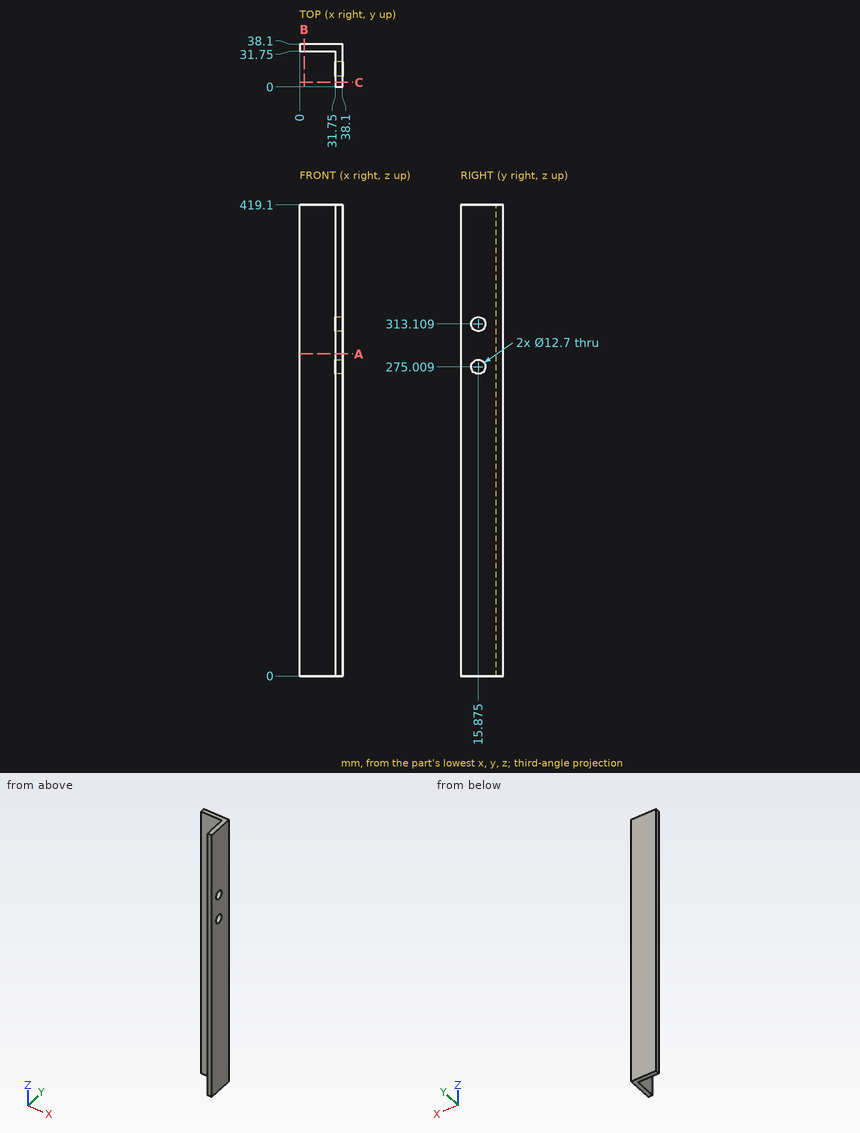
Answer from the drawing. Dimensions are ordinates in mm from the lowest x, y and z of the part. Round coordinates to 2 decimals unless told otherwise and drop trailing zeros. Write each loop counter-clockwise with the first axis right and the second up, starting at its lowest first coordinate (ties: lowest second). Pieces come first, ordered by that corner, then holes. Notation, with made-up numbers: (3, -8.75) - (13, -8.75) arc R18 ccw to (13, -1.75) - close; hole circle Ø11 at (79.25, 31). An arc over 180 degrees is marked (long way). One line per item, written item: value.
Q1. Find section A-A (z = 286.5). Determine the outline of the cut face in (x, y).
The answers:
outline: (0, 31.75) - (31.75, 31.75) - (31.75, 0) - (38.1, 0) - (38.1, 38.1) - (0, 38.1) - close
Q2. Each of these flat-tipped pins is pushed along its axis until it touches: P1, Ø5, axis at y = 16, z = 189, coming from the -X side; P2, Ø16, axis at x = 9, z = 312.5, coming from the -Y side. Where does it stop, or does it pass through?
The answers:
P1: stops at x = 31.75
P2: stops at y = 31.75
Q3. A straight line is drawn through the part: line 1 (X direction, y = 17.5, z = 62). Find the intervals that lie inside material, in ascending order. Write a range as from..to.
The answers:
line 1: x = 31.75..38.1
Q4. Find section B-B (x = 4). Determine the outline of the cut face in (y, z), and give its area (3 significant figures).
The answers:
outline: (31.75, 0) - (38.1, 0) - (38.1, 419.1) - (31.75, 419.1) - close
area: 2,660 mm2
